Model file for the job. Use its own axes, mm. Face numbers are marked on the shaded views. Round coordinates to 2 decimals unless told otherwise and drop trailing zeros. Loops run counter-clockwise (first coordinate to the right, second up) from the corner with the lowest first, then second, coordinate; pieces in that order, holes last. Notation, with made-up numbers: (13.25, 80) - (33.25, 80) arc R6 ccw to (33.25, 85) - close; hole circle Ø3 at (80.25, 49). An arc over 180 degrees is marked (long way). Answer as a JSON object with one key per item and string values.
from build123d import *

# Parameters (mm, degrees)
BOSS_EXTRUDE1_DEPTH      = 0.6
BOSS_EXTRUDE1_DEPTH_BACK = 0.6
SKETCH1_R                = 1.65
SKETCH2_W                = 8.1
SKETCH2_H                = 4.9
SKETCH2_W_2              = 6.7
SKETCH2_H_2              = 3.5
SKETCH2_W_3              = 22
SKETCH2_H_3              = 4.85
SKETCH2_W_4              = 20.6
SKETCH2_H_4              = 3.45
SKETCH2_W_5              = 4.7
SKETCH2_H_5              = 14
SKETCH2_W_6              = 3.3
SKETCH2_H_6              = 12.6
SKETCH2_H_7              = 10
SKETCH2_H_8              = 8.6
BOSS_EXTRUDE2_DEPTH      = 6
SKETCH3_W                = 9
SKETCH3_H                = 13.5
BOSS_EXTRUDE3_DEPTH      = 10.9
CUT_EXTRUDE1_DEPTH       = 10
SKETCH5_R                = 3.05
SKETCH5_R_2              = 0.75
CUT_EXTRUDE2_DEPTH       = 11.9
FILLET1_R                = 0.75


with BuildPart() as part:
    # Sketch1 → Boss-Extrude1 (new, two sides: drawn at the far end of the back side and taken through both)
    with BuildSketch(Plane(origin=(0, 0, 0), x_dir=(1, 0, 0), z_dir=(0, 1, 0)).offset(-BOSS_EXTRUDE1_DEPTH_BACK)):
        with BuildLine():
            Line((-67, 29.075), (67, 29.075))
            ThreePointArc((67, 29.075), (68.767766953, 28.342766953), (69.5, 26.575))
            Line((69.5, 26.575), (69.5, -26.575))
            ThreePointArc((69.5, -26.575), (68.767766953, -28.342766953), (67, -29.075))
            Line((67, -29.075), (-67, -29.075))
            ThreePointArc((-67, -29.075), (-68.767766953, -28.342766953), (-69.5, -26.575))
            Line((-69.5, -26.575), (-69.5, 26.575))
            ThreePointArc((-69.5, 26.575), (-68.767766953, 28.342766953), (-67, 29.075))
        make_face()
        with Locations(Location((-55.15, 20.075, 0), (0, 0, 270))):
            Circle(SKETCH1_R, mode=Mode.SUBTRACT)
        with Locations(Location((49.85, 20.075, 0), (0, 0, 270))):
            Circle(SKETCH1_R, mode=Mode.SUBTRACT)
        with Locations(Location((55.5, -8.075, 0), (0, 0, 270))):
            Circle(SKETCH1_R, mode=Mode.SUBTRACT)
        with Locations(Location((-56, -8.075, 0), (0, 0, 270))):
            Circle(SKETCH1_R, mode=Mode.SUBTRACT)
    extrude(amount=BOSS_EXTRUDE1_DEPTH + BOSS_EXTRUDE1_DEPTH_BACK)

    # Sketch2 → Boss-Extrude2 (add)
    # profile 1 of 4: a face of its own
    with BuildSketch(Plane(origin=(0, 0.6, 0), x_dir=(1, 0, 0), z_dir=(0, 1, 0))):
        with Locations((-62.45, 25.025)):
            Rectangle(SKETCH2_W, SKETCH2_H)
        with Locations((-62.45, 25.025)):
            Rectangle(SKETCH2_W_2, SKETCH2_H_2, mode=Mode.SUBTRACT)
    # profile 2 of 4: a face of its own
    with BuildSketch(Plane(origin=(0, 0.6, 0), x_dir=(1, 0, 0), z_dir=(0, 1, 0))):
        with Locations((-34.15, 25.4)):
            Rectangle(SKETCH2_W_3, SKETCH2_H_3)
        with Locations((-34.15, 25.4)):
            Rectangle(SKETCH2_W_4, SKETCH2_H_4, mode=Mode.SUBTRACT)
    # profile 3 of 4: a face of its own
    with BuildSketch(Plane(origin=(0, 0.6, 0), x_dir=(1, 0, 0), z_dir=(0, 1, 0))):
        with Locations((-66.15, -8.825)):
            Rectangle(SKETCH2_W_5, SKETCH2_H_5)
        with Locations((-66.15, -8.825)):
            Rectangle(SKETCH2_W_6, SKETCH2_H_6, mode=Mode.SUBTRACT)
    # profile 4 of 4: a face of its own
    with BuildSketch(Plane(origin=(0, 0.6, 0), x_dir=(1, 0, 0), z_dir=(0, 1, 0))):
        with Locations((66.65, -7.075)):
            Rectangle(SKETCH2_W_5, SKETCH2_H_7)
        with Locations((66.65, -7.075)):
            Rectangle(SKETCH2_W_6, SKETCH2_H_8, mode=Mode.SUBTRACT)
    extrude(amount=BOSS_EXTRUDE2_DEPTH)

    # Sketch3 → Boss-Extrude3 (add)
    with BuildSketch(Plane(origin=(0, 0.6, 0), x_dir=(1, 0, 0), z_dir=(0, 1, 0))):
        with Locations((-62.4, -24.325)):
            Rectangle(SKETCH3_W, SKETCH3_H)
    extrude(amount=BOSS_EXTRUDE3_DEPTH)

    # Sketch4 → Cut-Extrude1 (cut)
    with BuildSketch(Plane(origin=(0, 0, 17.575), x_dir=(-1, 0, 0), z_dir=(0, 0, -1))):
        with BuildLine():
            Line((57.9, 11.5), (57.9, 7))
            ThreePointArc((57.9, 7), (59.218019485, 10.181980515), (62.4, 11.5))
            Line((62.4, 11.5), (57.9, 11.5))
        make_face()
        with BuildLine():
            Line((66.9, 11.5), (62.4, 11.5))
            ThreePointArc((62.4, 11.5), (65.581980515, 10.181980515), (66.9, 7))
            Line((66.9, 7), (66.9, 11.5))
        make_face()
    extrude(amount=-CUT_EXTRUDE1_DEPTH, mode=Mode.SUBTRACT)

    # Sketch5 → Cut-Extrude2 (cut)
    with BuildSketch(Plane.XY.offset(31.075)):
        with Locations((-62.4, 7.1)):
            Circle(SKETCH5_R)
        with Locations((-62.4, 7.1)):
            Circle(SKETCH5_R_2, mode=Mode.SUBTRACT)
    extrude(amount=-CUT_EXTRUDE2_DEPTH, mode=Mode.SUBTRACT)

    # Fillet1
    fillet1_edges = [part.edges().sort_by_distance(p)[0] for p in [
        (-63.15, 7.1, 31.075),
    ]]
    fillet(fillet1_edges, radius=FILLET1_R)


solid = part.part
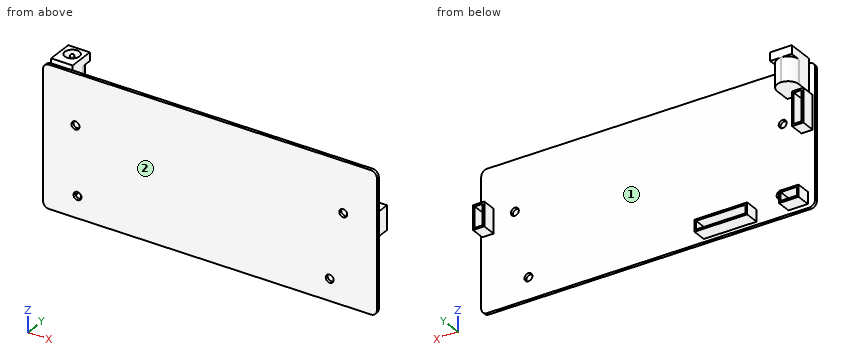
1) Slice it at B-B on z = -20.5. List the corners of the cut face in (x, y).
Values follow:
{"outline": "(-69.5, -0.6) - (-56.74, -0.6) - (-56.74, 0.6) - (-69.5, 0.6) - close; (-53.56, -0.6) - (48.26, -0.6) - (48.26, 0.6) - (-53.56, 0.6) - close; (51.44, -0.6) - (69.5, -0.6) - (69.5, 0.6) - (51.44, 0.6) - close"}
2) Slice it at C-C on z = -8. List the corners of the cut face in (x, y), then the cut area to 3 significant figures.
Values follow:
{"outline": "(-69.5, -0.6) - (69.5, -0.6) - (69.5, 0.6) - (-69.5, 0.6) - close", "area": "167 mm²"}
3) Drop flat-ended pins along their axis: P1, Ø6.5, axis at y = 5, z = 5, coming from the +X side; P2, Ø1.8, axis at x = -62, z = -24.5, coming from the +Y side; P3, Ø4, axis at y = 4.5, z = -21.5, coming from the -X side; P4, Ø4, axis at x = 45, y = 3, coming from the -Z side. Give the stop position or say it passes through.
Values follow:
{"P1": "x = 69", "P2": "y = 0.6", "P3": "x = -66.5", "P4": "through"}
4) Two-plate mould, pull along X, no slides. Class the marked faces 1 and 2: pulls with the +X half, pulls with the -X half, needs draft (parallel to the pull), parting line crosses it, or undercut.
Values follow:
{"face 1": "undercut", "face 2": "needs draft"}
5) Slice it at A-A on x = 49.85. List the corners of the cut face in (y, z) (3 decimals).
Values follow:
{"outline": "(-0.6, -29.075) - (0.6, -29.075) - (0.6, -21.725) - (-0.6, -21.725) - close; (-0.6, -18.425) - (0.6, -18.425) - (0.6, 29.075) - (-0.6, 29.075) - close"}
6) Slice it at D-D on x = 24. List the corners of the cut face in (y, z) (3 decimals).
Values follow:
{"outline": "(-0.6, -29.075) - (0.6, -29.075) - (0.6, 29.075) - (-0.6, 29.075) - close"}
7) Probe probe 1 along Z at (x, y) = (-35, 1.25) (3 decimals); probe 2 along X at (y, z) = (3.5, 12.5); probe 3 along Y at (x, z) = (29, 4). List the from-to ranges inside material, lowest first.
Values follow:
{"probe 1": "-27.825 to -27.125, -23.675 to -22.975", "probe 2": "-68.5 to -67.8, -64.5 to -63.8", "probe 3": "-0.6 to 0.6"}
